```python
from build123d import *

# Parameters (mm, degrees)
SKETCH1_W           = 9
SKETCH1_H           = 11
BOSS_EXTRUDE1_DEPTH = 3.3
BOSS_EXTRUDE2_DEPTH = 10.3


with BuildPart() as part:
    # Sketch1 → Boss-Extrude1 (new body)
    with BuildSketch(Plane.XY):
        Rectangle(SKETCH1_W, SKETCH1_H)
    extrude(amount=BOSS_EXTRUDE1_DEPTH)

    # Sketch2 → Boss-Extrude2 (add)
    with BuildSketch(Plane(origin=(0, 0, 0), x_dir=(-1, 0, 0), z_dir=(0, 0, -1))):
        with BuildLine():
            Line((-4.5, 1), (-4.5, -5.5))
            Line((-4.5, -5.5), (4.5, -5.5))
            Line((4.5, -5.5), (4.5, 1))
            ThreePointArc((4.5, 1), (0, 5.5), (-4.5, 1))
        make_face()
    extrude(amount=BOSS_EXTRUDE2_DEPTH)


solid = part.part
```
Input: part model. Units: mm. Frame: model coordinates. A direction names the side the tool comes from. Round coordinates to 2 decimals unless told otherwise and drop trailing zeros. Loops run counter-clockwise (first coordinate to the right, second up) from the corner with the lowest first, then second, coordinate; pieces in that order, holes last. Notation, with made-up numbers: (7.5, 45) -> (65.5, 45) arc R25 ccw to (65.5, 72) -> close; hole circle Ø9 at (-31.5, -36). An arc over 180 degrees is marked (long way). One line per item, written item: value.
(1) Mould query, pull axis X, two halves, no side actions, for faces 1 (the face through (3, 5, 0)), 2 (the face through (-0.1, 5.5, -5.1)), 3 (the face through (4.5, -1, -2)). Classes: pulls with the +X half, pulls with the -X half, needs draft (parallel to the pull), parting line crosses it, or undercut.
Geometry check:
face 1: needs draft
face 2: parting line crosses it
face 3: pulls with the +X half
(2) Material intervals for line 1 (Z direction, x = 3.75, y = 4.5); line 2 (X direction, y = 2.5, z = -9); line 3 (Y direction, x = -3.25, z = -8.25), sorted ascending. Write a range as [from, to].
Geometry check:
line 1: [0, 3.3]
line 2: [-4.24, 4.24]
line 3: [-5.5, 4.11]
(3) Section B-B (y = 3.75). Return the cut outline in (x, z), plus the area to 3 significant figures.
Geometry check:
outline: (-4.5, 0) -> (-3.56, 0) -> (-3.56, -10.3) -> (3.56, -10.3) -> (3.56, 0) -> (4.5, 0) -> (4.5, 3.3) -> (-4.5, 3.3) -> close
area: 103 mm2
(4) Set-up query: faces 4 (the face through (-4, 4, 0)), 5 (the face through (0, 0, 3.3)). Return all of +Z, -Z, +X, -X, +Y, -Y with unobstructed straight access to the full face (end or side cutting, diameter ignored); none if empty.
Geometry check:
face 4: -Z, -X, +Y
face 5: +Z, +X, -X, +Y, -Y
(5) Section C-C (x = 2.25). Return the cut outline in (y, z), plus the area to 3 significant figures.
Geometry check:
outline: (-5.5, -10.3) -> (4.9, -10.3) -> (4.9, 0) -> (5.5, 0) -> (5.5, 3.3) -> (-5.5, 3.3) -> close
area: 143 mm2
(6) Section D-D (y = 2.25). Return the cut outline in (x, z), plus the area to 3 significant figures.
Geometry check:
outline: (-4.5, 0) -> (-4.32, 0) -> (-4.32, -10.3) -> (4.32, -10.3) -> (4.32, 0) -> (4.5, 0) -> (4.5, 3.3) -> (-4.5, 3.3) -> close
area: 119 mm2
(7) Section A-A (z = -7.5). Return the cut outline in (x, y).
Geometry check:
outline: (-4.5, -5.5) -> (4.5, -5.5) -> (4.5, 1) arc R4.5 ccw to (-4.5, 1) -> close
(8) Pin query (flat end, axial travel): pin 1 (1.5 mm diameter, centred on y = 3.5, z = -4.5, fed in from +X). Return the tip coordinate at first contact, or that it passes through.
Geometry check:
pin 1: x = 4.15
